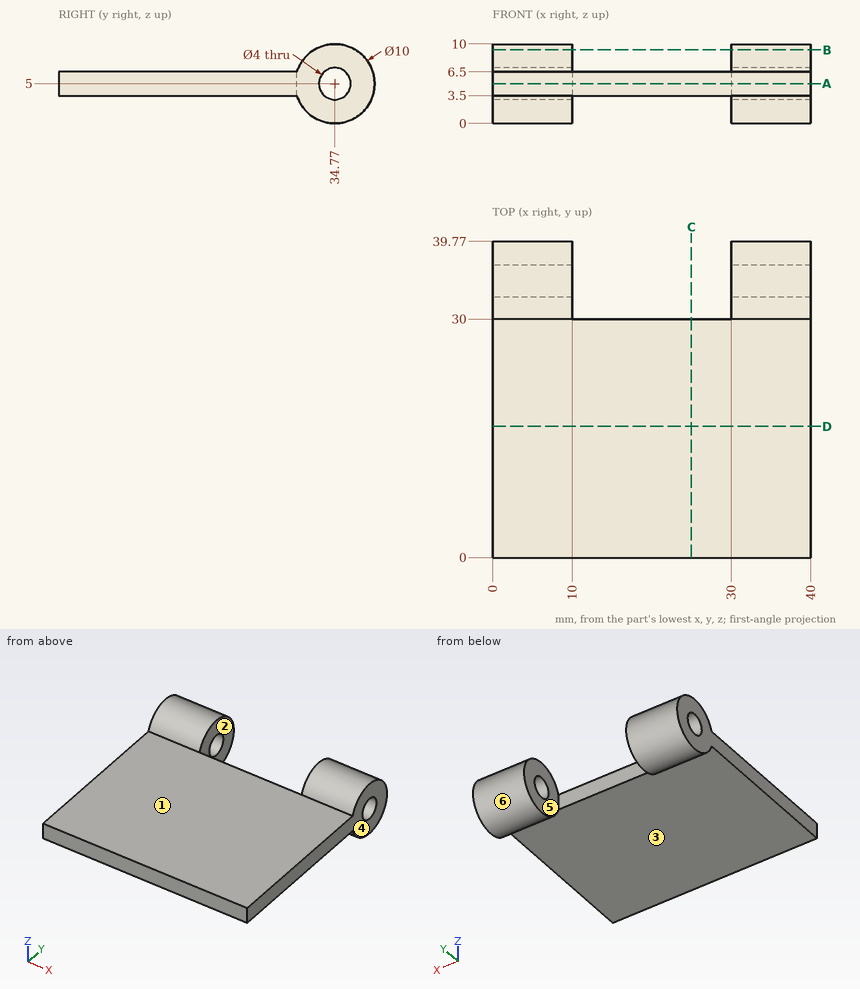
The drawing under review shows one solid part. Ordinate dimensions are in mm from its lowest x, y, z. A direction names the side the tool comes from. Round coordinates to 2 decimals unless told otherwise and drop trailing zeros. Write each loop counter-clockwise with the first axis right and the second up, starting at its lowest first coordinate (ties: lowest second). Pieces come first, ordered by that corner, then holes.
(1) We need section C-C on x = 25. Give the boundary of the cut face in (y, z), and give its area (3 significant figures).
(2) Insertion check: pin 1 (4 mm diameter, centred on x = 16, y = 31.5, fed in from +Z); pin 2 (3.5 mm diameter, centred on x = 15, z = 5, fed in from +Y); pin 3 (4 mm diameter, centred on x = 16.5, y = 10, fed in from -Z). Each pin has a flat end and moves straight along its axis. Give the tip position at first contact, or say it passes through.
(3) We need section B-B on z = 9.25. Give the boundary of the cut face in (x, y).
(4) Wall thickness on L1, parallel to Y at x = 32.75, z = 5; L2, parallel to X at y = 37, z = 4; L3, parallel to Z at x = 28.5, y = 16.5: over which ranges is each line inside the solid? List them lowest first.
(5) Machinability: for the marked faces 1, 2 and 3, which of the approach directions +Z, -Z, +X, -X, +Y, -Y give a long, thin tool a straight path to every point of the face, cutting with its end or side? Answer none if there is none.
(6) We need section A-A on z = 5. Give the boundary of the cut face in (x, y), and give its area (3 significant figures).
(7) We need section D-D on y = 16.5. Give the boundary of the cut face in (x, z), and give its area (3 significant figures).
(8) Mouldability with a two-part tool opening along X and no side actions: class the marked faces 4, 5 and 6 as +X half, -X half, draft (parallel to the pull), parting line (faces both ways), or undercut.
Findings below:
1. outline: (0, 3.5) - (30, 3.5) - (30, 6.5) - (0, 6.5) - close
1. area: 90.0 mm2
2. pin 1: stops at z = 6.5
2. pin 2: stops at y = 30
2. pin 3: stops at z = 3.5
3. outline: (0, 32.14) - (10, 32.14) - (10, 37.4) - (0, 37.4) - close; (30, 32.14) - (40, 32.14) - (40, 37.4) - (30, 37.4) - close
4. L1: y = 0 to 32.77, 36.77 to 39.77
4. L2: x = 0 to 10, 30 to 40
4. L3: z = 3.5 to 6.5
5. face 1: +Z, +X, -X, -Y
5. face 2: +Z, -Z, +Y
5. face 3: -Z, +X, -X, -Y
6. outline: (0, 0) - (40, 0) - (40, 32.77) - (30, 32.77) - (30, 30) - (10, 30) - (10, 32.77) - (0, 32.77) - close; (0, 36.77) - (10, 36.77) - (10, 39.77) - (0, 39.77) - close; (30, 36.77) - (40, 36.77) - (40, 39.77) - (30, 39.77) - close
6. area: 1,320 mm2
7. outline: (0, 3.5) - (40, 3.5) - (40, 6.5) - (0, 6.5) - close
7. area: 120 mm2
8. face 4: +X half
8. face 5: undercut
8. face 6: draft
